Could you check a few things on this model? Use its own coordinates, in mm. Round coordinates to 2 decimals unless told otherwise and drop trailing zeros. Loops run counter-clockwise (first coordinate to the right, second up) from the corner with the lowest first, then second, coordinate; pieces in that order, holes last. Notation, with made-up numbers: (89.5, -38.75) - (135.5, -38.75) arc R6 ccw to (135.5, -28.75) - close; hole circle Ø3 at (15, 69.25). An arc over 180 degrees is marked (long way). Answer as CSV lines item,"result". Start each with the question number.
1) We'd pull the mould along Z, two halves only. Please class faces 1 (the face through (-5, 1, -12.5)), 2 (the face through (-4.87, 0.79, -8.49)), 3 (the face through (-5, 1.6, -6)): pulls with the +Z half, pulls with the -Z half, needs draft (parallel to the pull), parting line crosses it, or undercut.
2) Suppose I cut it at C-C, the plane y = 0.25. Write out the boundary of the cut face in (x, z), then the cut area to 3 significant figures.
3) Suppose I cut it at D-D, the plane z = -7.5. Write out the boundary of the cut face in (x, y), then the cut area to 3 significant figures.
4) Suppose I cut it at B-B, the plane x = -5. Write out the boundary of the cut face in (y, z), then the cut area to 3 significant figures.
5) Suppose I cut it at A-A, the plane z = -5. Write out the boundary of the cut face in (x, y), then the cut area to 3 significant figures.
6) Please list where this line runs through material, in increasing order: line 1 along Z through (x, y) = (-5, 1.4).
Autodesk Inventor part; units mm, degrees
ref_plane "YZ Plane" through (0, 0, 0) normal (1, 0, 0) x (0, 1, 0)
ref_plane "XZ Plane" through (0, 0, 0) normal (0, 1, 0) x (-1, 0, 0)
ref_plane "XY Plane" through (0, 0, 0) normal (0, 0, 1) x (1, 0, 0)
sketch "Sketch1" plane through (0, 0, 0) normal (0, 1, 0) x (-1, 0, 0)
  line L0 (0, 0) -> (10, 0)
  line L1 (10, 0) -> (10, -12.5)
  line L2 (10, -12.5) -> (0, -12.5)
  line L3 (0, -12.5) -> (0, 0)
  line L4 (5, -3.5761) -> (5, -9.8666) construction
  circle A0 centre (5, -5) radius 0.75
  circle A1 centre (5, -7.5) radius 1
  dimension "d0" = 10
  dimension "d1" = 12.5
  dimension "d2" = 7.5
  dimension "d3" = 7.5
  dimension "d6" = 1.5
  dimension "d7" = 2
extrude "Extrusion1" add sketch "Sketch1" along normal blind 1.6
properties part number "Slit_insert"
Filled sheet:
1,face 1,"pulls with the -Z half"
1,face 2,"undercut"
1,face 3,"needs draft"
2,outline,"(-10, -12.5) - (0, -12.5) - (0, 0) - (-10, 0) - close; hole circle Ø2 at (-5, -7.5); hole circle Ø1.5 at (-5, -5)"
2,area,"120 mm²"
3,outline,"(-10, 0) - (-6, 0) - (-6, 1.6) - (-10, 1.6) - close; (-4, 0) - (0, 0) - (0, 1.6) - (-4, 1.6) - close"
3,area,"12.8 mm²"
4,outline,"(0, -12.5) - (1.6, -12.5) - (1.6, -8.5) - (0, -8.5) - close; (0, -6.5) - (1.6, -6.5) - (1.6, -5.75) - (0, -5.75) - close; (0, -4.25) - (1.6, -4.25) - (1.6, 0) - (0, 0) - close"
4,area,"14.4 mm²"
5,outline,"(-10, 0) - (-5.75, 0) - (-5.75, 1.6) - (-10, 1.6) - close; (-4.25, 0) - (0, 0) - (0, 1.6) - (-4.25, 1.6) - close"
5,area,"13.6 mm²"
6,line 1,"-12.5 to -8.5, -6.5 to -5.75, -4.25 to 0"
